from build123d import *

# Parameters (mm, degrees)
SKETCH_1_W          = 65
SKETCH_1_H          = 68
SKETCH_1_R          = 21
SKETCH_1_R_2        = 2.6
EXTRUDE_1_DEPTH     = 3
SKETCH_2_W          = 65
SKETCH_2_H          = 3
EXTRUDE_2_DEPTH     = 65
CUT_EXTRUDE_1_DEPTH = 65
FILLET_1_R          = 3


with BuildPart() as part:
    # 草图1 → 凸台-拉伸1 (new body)
    with BuildSketch(Plane.XY):
        Rectangle(SKETCH_1_W, SKETCH_1_H)
        with Locations((0, 5)):
            Circle(SKETCH_1_R, mode=Mode.SUBTRACT)
        with Locations((23.5, 28.5)):
            Circle(SKETCH_1_R_2, mode=Mode.SUBTRACT)
        with Locations((-23.5, 28.5)):
            Circle(SKETCH_1_R_2, mode=Mode.SUBTRACT)
        with Locations((-23.5, -18.5)):
            Circle(SKETCH_1_R_2, mode=Mode.SUBTRACT)
        with Locations((23.5, -18.5)):
            Circle(SKETCH_1_R_2, mode=Mode.SUBTRACT)
    extrude(amount=EXTRUDE_1_DEPTH)

    # 草图2 → 凸台-拉伸2 (add)
    with BuildSketch(Plane.XY.offset(3)):
        with Locations((0, -32.5)):
            Rectangle(SKETCH_2_W, SKETCH_2_H)
    extrude(amount=EXTRUDE_2_DEPTH)

    # 草图3 → 切除-拉伸1 (cut)
    with BuildSketch(Plane(origin=(0, -31, 0), x_dir=(1, 0, 0), z_dir=(0, 1, 0))):
        with BuildLine():
            Line((22, -16), (22, -58))
            ThreePointArc((22, -58), (19.9, -60.1), (17.8, -58))
            Line((17.8, -58), (17.8, -16))
            ThreePointArc((17.8, -16), (19.9, -13.9), (22, -16))
        make_face()
        with BuildLine():
            Line((-22, -16), (-22, -58))
            ThreePointArc((-22, -58), (-19.9, -60.1), (-17.8, -58))
            Line((-17.8, -58), (-17.8, -16))
            ThreePointArc((-17.8, -16), (-19.9, -13.9), (-22, -16))
        make_face()
    extrude(amount=-CUT_EXTRUDE_1_DEPTH, mode=Mode.SUBTRACT)

    # 圆角1
    fillet_1_edges = [part.edges().sort_by_distance(p)[0] for p in [
        (0, -34, 0),
    ]]
    fillet(fillet_1_edges, radius=FILLET_1_R)


solid = part.part
Source: CAD feature listing. Evaluate the final solid. Frame: model axes, mm. A direction names the side the tool comes from. Coordinates: 2 decimals unless noted, no trailing zeros. Order: outer loops, then holes, each group sorted by start corner. A loop starts at its lowest first (then second) coordinate and runs counter-clockwise, first axis right, second up. Notation, with made-up numbers: M 39.25,69 L 54.25,69 A12 cw 54.25,84 Z; hole C 88,-3 d3. An arc over 180 degrees is marked long. Write each question's results on one line, items separated by ' | '. Start each with the question number.
1. Section C-C, the plane x = -1. Return the cut outline in (y, z), then the cut area to 3 significant figures.
2. Section A-A, the plane z = 52. Return the cut outline in (x, y).
3. Section D-D, the plane x = -23.5. Return the cut outline in (y, z), then the cut area to 3 significant figures.
4. Pin query (flat end, axial travel): pin 1 (6 mm diameter, centred on x = 23.5, y = 28.5, fed in from +Z); pin 2 (12 mm diameter, centred on x = -6.5, z = 22.5, fed in from +Y); pin 3 (5 mm diameter, centred on x = -3, y = 21, fed in from +Z); pin 4 (12 mm diameter, centred on x = -17.5, y = 24.5, fed in from -Z). Return the tip coordinate at first contact, or that it passes through.
5. Material intervals for L1, parallel to Y at x = -23, z = 1; L2, parallel to X at y = -18, z = 1; L3, parallel to Y at x = 23.5, z = 0.8, sorted ascending.
6. Reachability of faces 1 (the face through (24.9, 30.69, 1.48)), 2 (the face through (0, -31, 35)), 3 (the face through (-19.9, -32.5, 60.1)) from +Z, -Z, +X, -X, +Y, -Y: full face, straight path, thin tool, end or side. Return the list, or none.
7. Section B-B, the plane y = 28.5. Return the cut outline in (x, z), then the cut area to 3 significant figures.
8. Draft query along Z for faces 4 (the face through (19.9, -32.5, 60.1)), 5 (the face through (25.98, -17.72, 1.48)), 6 (the face through (-15, -12, 3)). Return one class per face: +Z half, -Z half, draft (parallel to the pull), parting line (faces both ways), or undercut.
Solution:
1) outline: M -34,3 A3 ccw -31,0 L -15.98,0 L -15.98,3 L -31,3 L -31,68 L -34,68 Z; M 25.98,0 L 34,0 L 34,3 L 25.98,3 Z | area: 271 mm²
2) outline: M -32.5,-34 L -22,-34 L -22,-31 L -32.5,-31 Z; M -17.8,-34 L 17.8,-34 L 17.8,-31 L -17.8,-31 Z; M 22,-34 L 32.5,-34 L 32.5,-31 L 22,-31 Z
3) outline: M -34,3 A3 ccw -31,0 L -21.1,0 L -21.1,3 L -31,3 L -31,68 L -34,68 Z; M -15.9,0 L 25.9,0 L 25.9,3 L -15.9,3 Z; M 31.1,0 L 34,0 L 34,3 L 31.1,3 Z | area: 366 mm²
4) pin 1: z = 3 | pin 2: y = -31 | pin 3: through | pin 4: z = 0
5) L1: -33.24 to -21.05, -15.95 to 25.95, 31.05 to 34 | L2: -32.5 to -26.05, -20.95 to 20.95, 26.05 to 32.5 | L3: -33.04 to -21.1, -15.9 to 25.9, 31.1 to 34
6) face 1: +Z, -Z | face 2: +Z, +X, -X, +Y | face 3: +Y, -Y
7) outline: M -32.5,0 L -26.1,0 L -26.1,3 L -32.5,3 Z; M -20.9,0 L 20.9,0 L 20.9,3 L -20.9,3 Z; M 26.1,0 L 32.5,0 L 32.5,3 L 26.1,3 Z | area: 164 mm²
8) face 4: undercut | face 5: draft | face 6: +Z half
